Input: part model. Units: mm. Frame: model coordinates. A direction names the side the tool comes from. Give positions to 0.01 mm unless a question says otherwise; leave off trailing zeros. Loops run counter-clockwise (first coordinate to the right, second up) from the corner with the lowest first, then second, coordinate; pieces in that order, holes last. Notation, with made-up numbers: M 12.25,-37 L 34.25,-37 A19 cw 34.25,-17 Z; hole C -21.5,45.5 d4. An arc over 180 degrees is marked long. One line per item, written item: value. Start each with the question number.
(1) Access query for faces 4 (the cylindrical face through (2485.2, 4693.96, 2.46)), 5 (the flat face through (2468.808, 4724, 2)), 6 (the flat face through (2481.808, 4725, 2)). Directions: +Z, -Z, +X, -X, +Y, -Y. A direction counts if a zero-diameter tool reaches every point of the face in a straight line with its end or side. Return the directions, or none.
(2) Pull-direction query (Y, two-part tool) for faces 1 (the flat face through (2472, 4704, 5)), 2 (the flat face through (2475, 4742.948, 2)), 3 (the cylindrical face through (2474.2, 4682.96, 2.46)); classes: released by +Y, released by -Y, zero draft, split by the parting line, or undercut.
(3) Ray query, line 1 along X through (y, z) = (4729.5, 2.7); line 2 along X through (y, z) = (4682, 4.65); line 3 along X through (y, z) = (4704.5, 4.1). Return the intervals inside material, ascending. Write a range as from..to.
(4) Section C-C on y = 4712. Output: boundary loops of the cut face in (x, z).
(5) Section A-A on z = 4. Output: boundary loops of the cut face in (x, y), plus the area to 3 significant figures.
(6) Pin query (flat end, axial travel): P1, Ø1.8, axis at x = 2464.31, y = 4692.95, coming from the +Z side; P2, Ø1, axis at y = 4727, z = 3, coming from the -X side; P3, Ø1.5, axis at y = 4707, z = 3.5, coming from the +X side; P4, Ø2, axis at x = 2473, z = 1.5, coming from the -Y side. Return the tip coordinate at first contact, or that it passes through.
(7) Section B-B on x = 2465. Output: boundary loops of the cut face in (y, z) (3 decimals), plus the area to 3 significant figures.
```python
from build123d import *

# Parameters (mm, degrees)
SKETCH_1_R      = 1.5
EXTRUDE_1_DEPTH = 5


with BuildPart() as part:
    # 草图1 → 凸台-拉伸1 (new body)
    with BuildSketch(Plane.XY):
        with BuildLine():
            Line((2468.807860146, 4706.466341516), (2468.807860146, 4742.947835682))
            Line((2468.807860146, 4742.947835682), (2481.807860146, 4742.947835682))
            Line((2481.807860146, 4742.947835682), (2481.807860146, 4706.466341516))
            ThreePointArc((2481.807860146, 4706.466341516), (2475.307860146, 4677.947835682), (2468.807860146, 4706.466341516))
        make_face()
        with Locations((2475.307860146, 4692.947835682)):
            Circle(SKETCH_1_R, mode=Mode.SUBTRACT)
        with Locations((2464.307860146, 4692.947835682)):
            Circle(SKETCH_1_R, mode=Mode.SUBTRACT)
        with Locations((2486.307860146, 4692.947835682)):
            Circle(SKETCH_1_R, mode=Mode.SUBTRACT)
        with Locations((2475.307860146, 4703.947835682)):
            Circle(SKETCH_1_R, mode=Mode.SUBTRACT)
        with Locations((2475.307860146, 4681.947835682)):
            Circle(SKETCH_1_R, mode=Mode.SUBTRACT)
    extrude(amount=EXTRUDE_1_DEPTH)


solid = part.part
```
Output values:
1. face 4: +Z, -Z
1. face 5: +Z, -Z, -X, +Y
1. face 6: +Z, -Z, +X, +Y
2. face 1: zero draft
2. face 2: released by +Y
2. face 3: undercut
3. line 1: x = 2468.81..2481.81
3. line 2: x = 2465.05..2473.81, 2476.81..2485.56
3. line 3: x = 2465.74..2473.91, 2476.7..2484.88
4. outline: M 2468.81,0 L 2481.81,0 L 2481.81,5 L 2468.81,5 Z
5. outline: M 2468.81,4706.47 A15 ccw long 2481.81,4706.47 L 2481.81,4742.95 L 2468.81,4742.95 Z; hole C 2464.31,4692.95 d3; hole C 2475.31,4681.95 d3; hole C 2475.31,4692.95 d3; hole C 2475.31,4703.95 d3; hole C 2486.31,4692.95 d3
5. area: 1,130 mm²
6. P1: passes through
6. P2: stops at x = 2468.81
6. P3: stops at x = 2482.24
6. P4: stops at y = 4678
7. outline: M 4682.051,0 L 4691.617,0 L 4691.617,5 L 4682.051,5 Z; M 4694.279,0 L 4703.845,0 L 4703.845,5 L 4694.279,5 Z
7. area: 95.7 mm²
